Geometry: final body of the model. Coordinates: model frame, mm. Give positions to 0.01 mm unless a question says otherwise; leave off trailing zeros. Loops run counter-clockwise (first coordinate to the right, second up) from the corner with the lowest first, then second, coordinate; pieces in that order, holes last. Notation, with made-up numbers: (83.5, -8) - (117.5, -8) arc R19 ccw to (117.5, 29) - close; hole circle Ø3 at (56.25, 3). An arc over 180 degrees is marked (long way). Use one line per item in the form item = value.
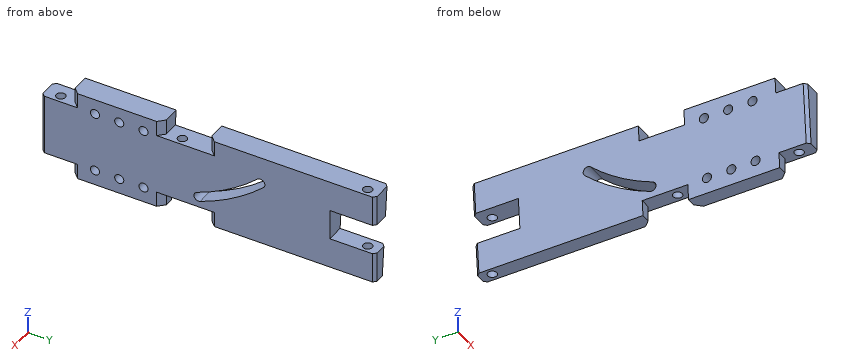
```python
from build123d import *

# Parameters (mm, degrees)
BOSS_EXTRUDE1_DEPTH = 19.05
SKETCH2_R           = 3.81
CUT_EXTRUDE1_DEPTH  = 64.5
SKETCH3_R           = 3.81
CUT_EXTRUDE2_DEPTH  = 64.5
CUT_EXTRUDE3_DEPTH  = 20.05
SKETCH6_R           = 3.81
CUT_EXTRUDE4_DEPTH  = 20.05
LPATTERN1_COUNT     = 3
LPATTERN1_PITCH     = 20.32
SKETCH7_W           = 25.4
SKETCH7_H           = 38.1
CUT_EXTRUDE5_DEPTH  = 20.05
CUT_EXTRUDE6_DEPTH  = 280.4
SKETCH9_R           = 3.81
CUT_EXTRUDE7_DEPTH  = 76.2
CHAMFER1_SIZE       = 2.54
CHAMFER2_SIZE       = 5.08


with BuildPart() as part:
    # Sketch1 → Boss-Extrude1 (new body)
    with BuildSketch(Plane(origin=(0, 0, 0), x_dir=(0, 0, -1), z_dir=(1, 0, 0))):
        Polygon((0, 0), (0, 25.4), (-12.7, 25.4), (-12.7, 101.6), (0, 101.6), (0, 139.7), (-12.7, 139.7), (-12.7, 279.4), (63.5, 279.4), (63.5, 139.7), (50.8, 139.7), (50.8, 101.6), (63.5, 101.6), (63.5, 25.4), (50.8, 25.4), (50.8, 0), align=None)
    extrude(amount=BOSS_EXTRUDE1_DEPTH)

    # Sketch2 → Cut-Extrude1 (cut, through all)
    with BuildSketch(Plane.XY):
        with Locations((12.7, 114.3)):
            Circle(SKETCH2_R)
    extrude(amount=-CUT_EXTRUDE1_DEPTH, mode=Mode.SUBTRACT)

    # Sketch3 → Cut-Extrude2 (cut, through all)
    with BuildSketch(Plane.XY):
        with Locations((12.7, 12.7)):
            Circle(SKETCH3_R)
    extrude(amount=-CUT_EXTRUDE2_DEPTH, mode=Mode.SUBTRACT)

    # Sketch4 → Cut-Extrude3 (cut, through all)
    with BuildSketch(Plane(origin=(19.05, 0, 0), x_dir=(0, 0, -1), z_dir=(1, 0, 0))):
        with BuildLine():
            ThreePointArc((45.433317408, 132.844708156), (31.8216378, 160.842664311), (13.115249698, 185.727085439))
            ThreePointArc((13.115249698, 185.727085439), (7.732489274, 185.968104562), (7.491470151, 180.585344138))
            ThreePointArc((7.491470151, 180.585344138), (25.319688182, 156.869120406), (38.292368451, 130.185526327))
            ThreePointArc((38.292368451, 130.185526327), (43.192433844, 127.944642763), (45.433317408, 132.844708156))
        make_face()
    extrude(amount=-CUT_EXTRUDE3_DEPTH, mode=Mode.SUBTRACT)

    # Sketch6 → Cut-Extrude4 (cut, through all)
    with BuildSketch(Plane(origin=(19.05, 0, 0), x_dir=(0, 0, -1), z_dir=(1, 0, 0))):
        with Locations((0, 44.904409269)):
            Circle(SKETCH6_R)
        with Locations((50.8, 44.904409269)):
            Circle(SKETCH6_R)
    cut_extrude4 = extrude(amount=-CUT_EXTRUDE4_DEPTH, mode=Mode.SUBTRACT)

    # LPattern1: Cut-Extrude4 ×3
    with Locations(*[(0, i * LPATTERN1_PITCH, 0) for i in range(1, LPATTERN1_COUNT)]):
        add(cut_extrude4, mode=Mode.SUBTRACT)

    # Sketch7 → Cut-Extrude5 (cut, through all)
    with BuildSketch(Plane(origin=(19.05, 0, 0), x_dir=(0, 0, -1), z_dir=(1, 0, 0))):
        with Locations((25.4, 260.35)):
            Rectangle(SKETCH7_W, SKETCH7_H)
    extrude(amount=-CUT_EXTRUDE5_DEPTH, mode=Mode.SUBTRACT)

    # Sketch8 → Cut-Extrude6 (cut, through all)
    with BuildSketch(Plane(origin=(0, 0, 0), x_dir=(1, 0, 0), z_dir=(0, 1, 0))):
        Polygon((0, 63.5), (6.666636161, 63.5), (0, -12.7), align=None)
    extrude(amount=CUT_EXTRUDE6_DEPTH, mode=Mode.SUBTRACT)

    # Sketch9 → Cut-Extrude7 (cut, symmetric)
    with BuildSketch(Plane.XY):
        with Locations((12.7, 269.24)):
            Circle(SKETCH9_R)
    extrude(amount=CUT_EXTRUDE7_DEPTH, both=True, mode=Mode.SUBTRACT)

    # Chamfer1
    chamfer1_edges = [part.edges().sort_by_distance(p)[0] for p in [
        (1.111106027, 279.4, 0),
        (5.555530134, 279.4, -50.8),
        (3.33331808, 0, -25.4),
        (19.05, 279.4, -50.8),
        (19.05, 0, -25.4),
        (19.05, 279.4, 0),
    ]]
    chamfer(chamfer1_edges, length=CHAMFER1_SIZE)

    # Chamfer2
    chamfer2_edges = [part.edges().sort_by_distance(p)[0] for p in [
        (19.05, 25.4, -57.15),
        (19.05, 101.6, -57.15),
        (19.05, 139.7, -57.15),
        (19.05, 139.7, 6.35),
        (19.05, 101.6, 6.35),
        (19.05, 25.4, 6.35),
    ]]
    chamfer(chamfer2_edges, length=CHAMFER2_SIZE)


solid = part.part
```
(1) Cut plane C-C (y = 183). Return the cut outline in (x, z), plus the area to 3 significant figures.
Solution:
outline = (0, 12.7) - (1.68, -6.5) - (19.05, -6.5) - (19.05, 12.7) - close; (2.47, -15.55) - (6.67, -63.5) - (19.05, -63.5) - (19.05, -15.55) - close
area = 1,040 mm2
(2) Cut plane A-A (y = 269.24). Return the cut outline in (x, z).
Solution:
outline = (0, 12.7) - (2.22, -12.7) - (8.89, -12.7) - (8.89, 12.7) - close; (4.44, -38.1) - (6.67, -63.5) - (8.89, -63.5) - (8.89, -38.1) - close; (16.51, -63.5) - (19.05, -63.5) - (19.05, -38.1) - (16.51, -38.1) - close; (16.51, -12.7) - (19.05, -12.7) - (19.05, 12.7) - (16.51, 12.7) - close
(3) Material intervals for L1, parallel to Y at x = 16, z = 5.5; L2, parallel to Y at x = 13.75, z = -52; L3, parallel to Y at x = 12.7, z = -26, sorted ascending. Write a range as from..to.
Solution:
L1 = 27.43..99.57, 141.73..267.34, 271.14..279.4
L2 = 25.4..41.29, 48.52..61.61, 68.84..81.93, 89.16..101.6, 139.7..265.58, 272.9..279.4
L3 = 0..8.89, 16.51..110.49, 118.11..155.75, 169.7..241.3
(4) Cut plane B-B (y = 12.7). Return the cut outline in (x, z).
Solution:
outline = (1.11, 0) - (5.56, -50.8) - (8.89, -50.8) - (8.89, 0) - close; (16.51, -50.8) - (19.05, -50.8) - (19.05, 0) - (16.51, 0) - close
(5) Pin query (flat end, axial travel): P1, Ø1, axis at x = 7, z = -45.5, coming from the +Y side; P2, Ø4, axis at x = 10.5, z = 4, coming from the -Y side; P3, Ø1, axis at y = 67.5, z = -1.5, coming from the +X side; P4, Ø2, axis at y = 110, z = -40.5, coming from the -X side. Return the tip coordinate at first contact, or that it passes through.
Solution:
P1 = 279.26
P2 = 25.4
P3 = through
P4 = 4.57
